Autodesk Inventor part; units mm, degrees
ref_plane "YZ Plane" through (0, 0, 0) normal (1, 0, 0) x (0, 1, 0)
ref_plane "XZ Plane" through (0, 0, 0) normal (0, 1, 0) x (-1, 0, 0)
ref_plane "XY Plane" through (0, 0, 0) normal (0, 0, 1) x (1, 0, 0)
sketch "Boceto1" plane through (0, 0, 0) normal (0, 0, 1) x (1, 0, 0)
  line L0 (-20, -20) -> (20, -20)
  line L1 (20, -20) -> (20, 20)
  line L2 (20, 20) -> (-20, 20)
  line L3 (-20, 20) -> (-20, -20)
  line L4 (-20, -20) -> (20, 20) construction
  line L5 (20, -20) -> (-20, 20) construction
  line L6 (-25, 25) -> (25, 25)
  line L7 (25, 25) -> (25, -25)
  line L8 (25, -25) -> (-25, -25)
  line L9 (-25, -25) -> (-25, 25)
  point P0 (0, 0)
  dimension "d0" = 40
  dimension "d1" = 40
  dimension "d2" = 5
extrude "Extrusión1" add sketch "Boceto1" against normal blind 6
extrude "Extrusión2" add sketch "Boceto1" along normal blind 2 contours L3 L2 L1 L0 | L6 L7 L8 L9
sketch "Boceto3" plane through (0, 0, 2) normal (0, 0, 1) x (1, 0, 0)
  line L0 (25, -25) -> (-25, -25)
  line L1 (-25, -25) -> (-25, 25)
  line L2 (-25, 25) -> (25, 25)
  line L3 (25, 25) -> (25, -25)
  line L4 (20, -20) -> (-20, -20)
  line L5 (-20, -20) -> (-20, 20)
  line L6 (-20, 20) -> (20, 20)
  line L7 (20, 20) -> (20, -20)
  line L8 (-20, -5) -> (20, -5) construction
  circle A0 centre (0, -5) radius 5
  circle A1 centre (0, -5) radius 6
  circle A2 centre (0, -5) radius 8
  line L9 (-20, 12) -> (20, 12) construction
  line L10 (0, 3) -> (0, -5) construction
  line L11 (5.5, 7) -> (-5.5, 7)
  line L12 (-7.5, 9) -> (-7.5, 15)
  line L13 (7.5, 15) -> (7.5, 9)
  line L14 (7.5, 7) -> (-7.5, 17) construction
  line L15 (-7.5, 7) -> (7.5, 17) construction
  line L16 (-3.9028, 17.8528) -> (-3.2066, 18.8472)
  line L17 (3.2066, 18.8472) -> (3.9028, 17.8528)
  line L18 (-1.5683, 19.7) -> (1.5683, 19.7)
  circle A3 centre (0, 12) radius 1.6258
  circle A4 centre (0, 12) radius 2.8258
  circle A5 centre (0, 12) radius 3.6258
  line L19 (-5.5, 17) -> (-5.5411, 17)
  line L20 (5.5411, 17) -> (5.5, 17)
  arc A6 (-5.5411, 17) -> (-3.9028, 17.8528) centre (-5.5411, 19) ccw
  arc A7 (-1.5683, 19.7) -> (-3.2066, 18.8472) centre (-1.5683, 17.7) ccw
  arc A8 (3.2066, 18.8472) -> (1.5683, 19.7) centre (1.5683, 17.7) ccw
  arc A9 (3.9028, 17.8528) -> (5.5411, 17) centre (5.5411, 19) ccw
  arc A10 (-5.5, 17) -> (-7.5, 15) centre (-5.5, 15) ccw
  arc A11 (-7.5, 9) -> (-5.5, 7) centre (-5.5, 9) ccw
  arc A12 (5.5, 7) -> (7.5, 9) centre (5.5, 9) ccw
  arc A13 (7.5, 15) -> (5.5, 17) centre (5.5, 15) ccw
  point P0 (0, 0)
  point P1 (-4.5, 17)
  point P2 (5.5206, 17)
  dimension "d13" = 15
  dimension "d14" = 10
  dimension "d17" = 1
  dimension "d18" = 2
  dimension "d21" = 9
  dimension "d22" = 15
  dimension "d23" = 10
  dimension "d25" = 3
  dimension "d27" = 3.2517
  dimension "d28" = 1.2
  dimension "d29" = 0.8
  dimension "d30" = 2.7
  dimension "d31" = 125
  dimension "d32" = 2
  dimension "d33" = 2
extrude "Extrusión4" cut sketch "Boceto3" against normal through all contours A0
extrude "Extrusión5" cut sketch "Boceto3" against normal blind 0.6 contours A2
extrude "Extrusión6" cut sketch "Boceto3" against normal blind 0.6 contours L11 A11 L12 A10 L19 A6 L16 A7 L18 A8 L17 A9 L20 A13 L13 A12 | A4
sketch "Boceto4" plane through (0, 0, -6) normal (0, 0, -1) x (-1, 0, 0)
  point P0 (0, 0)
equation "\"d1\" = d0"
equation "\"d14\" = D_camara"
equation "\"D_camara\" = 10"
properties part number "Tapa_camara"
Work out the finished part from the listing and answer in its coordinate system (mm). A direction names the side the tool comes from. Give positions to 0.01 mm unless a question says otherwise; leave off trailing zeros. Loops run counter-clockwise (first coordinate to the right, second up) from the corner with the lowest first, then second, coordinate; pieces in that order, holes last. Notation, with made-up numbers: M -14.5,16 L -0.5,16 A36 cw -0.5,51 Z; hole C 53.5,57.25 d9. An arc over 180 degrees is marked long. One line per item, written item: value. Start each with the question number.
1. Find section A-A (y = -5). Give the vertices of the cut face in (x, z), and give its area (3 significant figures).
2. Find section B-B (z = -0.75). Give the vertices of the cut face in (x, y).
3. Which of the six approach directions +Z, -Z, +X, -X, +Y, -Y give full straight-line access (tool end or side, diameter ignored) to faces 1 (the face through (0, -20, -3)), 2 (the face through (-1, 9, 2)), 3 (the face through (-6.93, 7.6, 1.7))?
4. Find section C-C (y = 12). Give the vertices of the cut face in (x, z), and give its area (3 significant figures).
5. Determine the mould class of faces 4 (the face through (0, -25, -2)), 5 (the face through (-4, -8, 1)), 6 (the face through (0, 25, -2)), 7 (the face through (0, 12, 2)) for opening direction Y: released by +Y, released by -Y, zero draft, split by the parting line, or undercut.
6. Find the intervals of material crossed by probe 1 along Y at (x, z) = (17, -4.5); probe 2 along Y at (x, z) = (0, 1.1), in increasing order.
7. Find section D-D (x = 12). Give the vertices of the cut face in (y, z).
8. This flat-tipped pin is pushed along its axis until it touches: P1, Ø1, axis at x = 5, y = -10, coming from the -Z side. Where does it stop, or does it pass through?
Reported:
1. outline: M -25,-6 L -20,-6 L -20,0 L -5,0 L -5,2 L -6,2 L -6,1.4 L -8,1.4 L -8,2 L -25,2 Z; M 5,0 L 20,0 L 20,-6 L 25,-6 L 25,2 L 8,2 L 8,1.4 L 6,1.4 L 6,2 L 5,2 Z
1. area: 138 mm²
2. outline: M -25,-25 L 25,-25 L 25,25 L -25,25 Z; hole M -20,-20 L 20,-20 L 20,20 L -20,20 Z
3. face 1: -Z
3. face 2: +Z, +X, -X, +Y, -Y
3. face 3: +Z
4. outline: M -25,-6 L -20,-6 L -20,0 L 20,0 L 20,-6 L 25,-6 L 25,2 L 7.5,2 L 7.5,1.4 L 3.63,1.4 L 3.63,2 L 2.83,2 L 2.83,1.4 L 1.63,1.4 L 1.63,2 L -1.63,2 L -1.63,1.4 L -2.83,1.4 L -2.83,2 L -3.63,2 L -3.63,1.4 L -7.5,1.4 L -7.5,2 L -25,2 Z
4. area: 154 mm²
5. face 4: released by -Y
5. face 5: undercut
5. face 6: released by +Y
5. face 7: zero draft
6. probe 1: y = -25 to -20, 20 to 25
6. probe 2: y = -25 to -10, 0 to 25
7. outline: M -25,-6 L -20,-6 L -20,0 L 20,0 L 20,-6 L 25,-6 L 25,2 L -25,2 Z
8. P1: stops at z = 0
